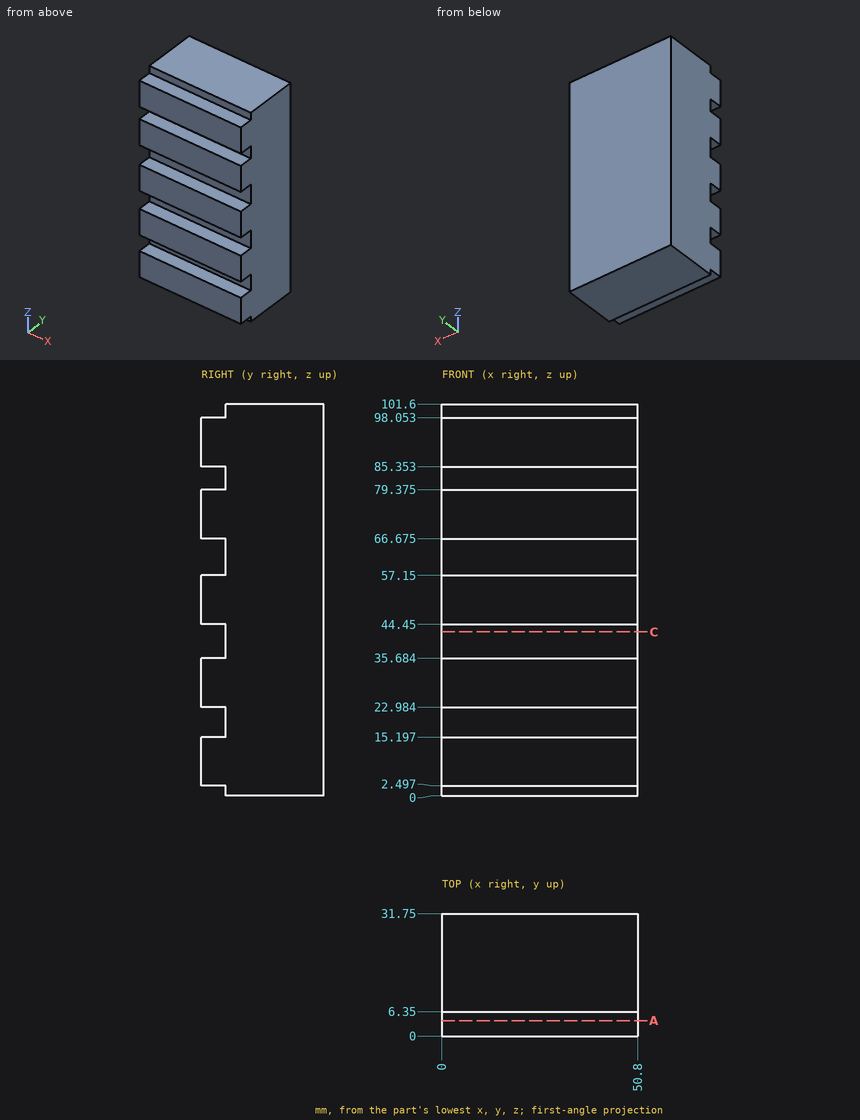
Here's the drawing with two shaded views (mm, measured from the low corner). I have some questions. Give positions to 0.01 mm unless a question says otherwise; leave off trailing zeros. Write each loop counter-clockwise with the first axis right and the second up, starting at its lowest first coordinate (ties: lowest second). Pieces come first, ordered by that corner, then holes. Notation, with made-up numbers: (-22, -37.75) -> (0, -37.75) arc R20 ccw to (0, -9.75) -> close; hole circle Ø8 at (55.25, -32). An arc over 180 degrees is marked (long way). Answer as a JSON object with one key per item and string values. Group by question number.
Item 1: I'm going to push flat-ended pins straight in: P1, Ø3, axis at x = 29.5, y = 1.5, coming from the +Z side; P2, Ø2.5, axis at x = 35.5, z = 20.5, coming from the -Y side; P3, Ø3, axis at x = 34.5, y = 2.5, coming from the -Z side. Where does each tip first touch, or does it pass through?
Item 2: Suppose I cut it at A-A (y = 4). State how many separate pieces and enclosed holes the cut face has, plus the area to 3 significant figures.
Item 3: Suppose I cut it at C-C (z = 42.5). Please give me the cut outline in (x, y).
Item 4: Please list where this line runs through material, in increasing order: line 1 (Y direction, x = 17, z = 83). Write a range as [from, to].
Findings:
{
 "1": {"P1": "stops at z = 98.05", "P2": "stops at y = 6.35", "P3": "stops at z = 2.5"},
 "2": {"separate pieces": "5", "enclosed holes": "0", "area": "3,230 mm²"},
 "3": {"outline": "(0, 6.35) -> (50.8, 6.35) -> (50.8, 31.75) -> (0, 31.75) -> close"},
 "4": {"line 1": "y = [6.35, 31.75]"}
}
